For this review, use the dimensioned drawing (mm, ordinates from the lowest corner) and the shaded views. Give positions to 0.01 mm unless a question says otherwise; leave off trailing zeros. Order: outer loops, then holes, each group sorted by start corner. A loop starts at its lowest first (then second) coordinate and runs counter-clockwise, first axis right, second up. Notation, with made-up numbers: (77.5, -35) -> (99.5, -35) arc R22 cw to (99.5, -27) -> close; hole circle Ø4 at (-27, 25). An arc over 180 degrees is marked (long way). Return JSON: item names as keys, results as strings.
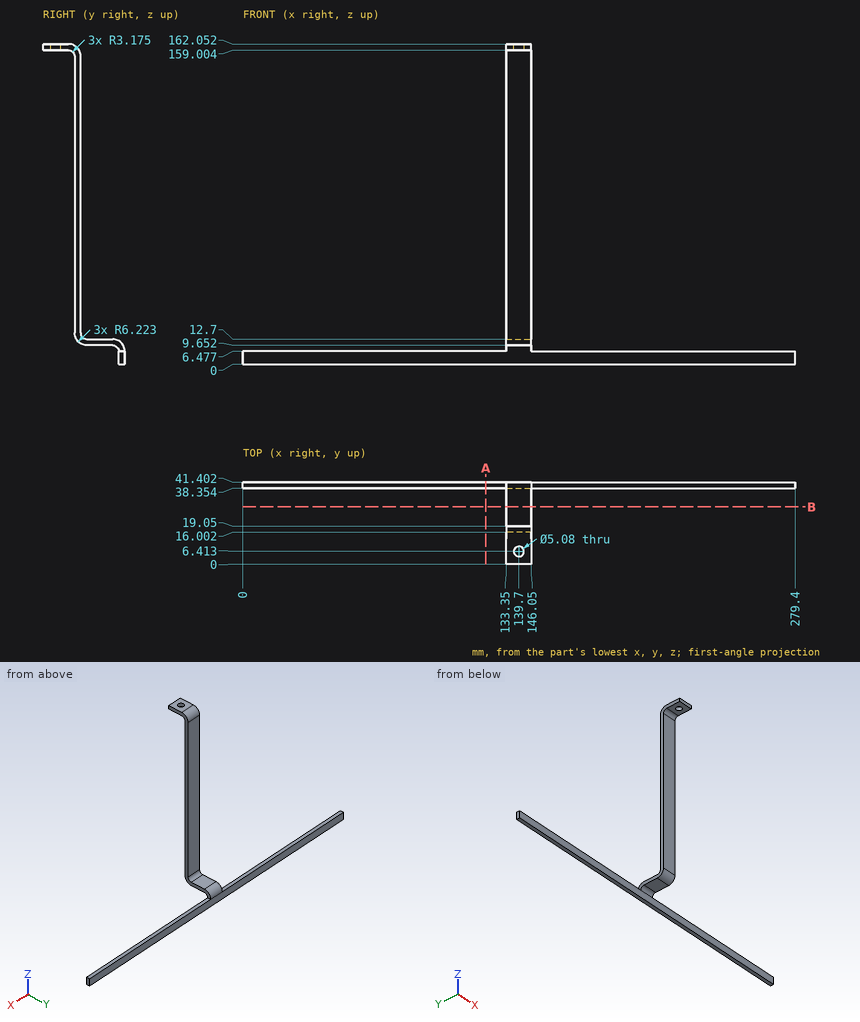
Item 1: Add section B-B (y = 29). Give the boundary of the cut face in (x, z), plus the area to 3 significant figures.
Result set:
{"outline": "(133.35, 9.65) -> (146.05, 9.65) -> (146.05, 12.7) -> (133.35, 12.7) -> close", "area": "38.7 mm^2"}
Item 2: For pin 1 (10 mm diameter, centred on x = 139, y = 30, fed in from +Z); pin 2 (2.5 mm diameter, centred on x = 228.5, y = 40, fed in from +Z); pin 3 (14 mm diameter, centred on x = 138, y = 27.5, fed in from -Z), all flat-tipped, find the tip position at first contact; note any pin that passes through.
Result set:
{"pin 1": "stops at z = 12.7", "pin 2": "stops at z = 6.48", "pin 3": "stops at z = 9.65"}
Item 3: Add section A-A (x = 123). Give the boundary of the cut face in (y, z) (1 decimal).
Result set:
{"outline": "(38.4, 0) -> (41.4, 0) -> (41.4, 6.5) -> (38.4, 6.5) -> close"}
Item 4: Wall thickness on L1, parallel to Y at x = 139.7, z = 160.3 (1 decimal); L2, parallel to Y at x = 139.7, z = 160.65 (1 decimal): over which ranges is each line inside the solid? List them lowest first. Write a range as [from, to].
Result set:
{"L1": "y = [0, 3.9], [9, 17.2]", "L2": "y = [0, 3.9], [9, 16.8]"}
